Check sheet for the modelled part. Datum: model origin and axes. Units: mm. Round coordinates to 2 decimals unless told otherwise and drop trailing zeros. Write each loop counter-clockwise with the first axis right and the second up, starting at its lowest first coordinate (ties: lowest second). Pieces come first, ordered by that corner, then holes. Notation, with made-up numbers: M 0.5,23 L 12.5,23 A37 ccw 12.5,60 Z; hole C -36,12.25 d9. An arc over 180 degrees is marked long. One line per item, written item: value.
from build123d import *

# Parameters (mm, degrees)
SKETCH1_R           = 1.483161667
BOSS_EXTRUDE1_DEPTH = 88.9
FILLET1_R           = 2.54


with BuildPart() as part:
    # Sketch1 → Boss-Extrude1 (new body)
    with BuildSketch(Plane.XY):
        Polygon((6.273667096, -0.450919823), (2.607492887, 5.899080177), (-4.724855532, 5.899080177), (-8.391029741, -0.450919823), (-4.724855532, -6.800919823), (2.607492887, -6.800919823), align=None)
        with Locations((-1.058681322, -0.450919823)):
            Circle(SKETCH1_R, mode=Mode.SUBTRACT)
    extrude(amount=BOSS_EXTRUDE1_DEPTH)

    # Fillet1
    fillet1_edges = [part.edges().sort_by_distance(p)[0] for p in [
        (2.607492887, -6.800919823, 44.45),
        (-4.724855532, -6.800919823, 44.45),
        (-8.391029741, -0.450919823, 44.45),
        (-4.724855532, 5.899080177, 44.45),
        (2.607492887, 5.899080177, 44.45),
        (6.273667096, -0.450919823, 44.45),
    ]]
    fillet(fillet1_edges, radius=FILLET1_R)


solid = part.part
Q1. Sectioned sample at B-B on z = 43. Enter the section's corners in (x, y).
Completed:
outline: M -7.66,-1.72 L -5.46,-5.53 A2.54 ccw -3.26,-6.8 L 1.14,-6.8 A2.54 ccw 3.34,-5.53 L 5.54,-1.72 A2.54 ccw 5.54,0.82 L 3.34,4.63 A2.54 ccw 1.14,5.9 L -3.26,5.9 A2.54 ccw -5.46,4.63 L -7.66,0.82 A2.54 ccw Z; hole C -1.06,-0.45 d2.97
Q2. Sectioned sample at D-D on x = 2.5. Enter the section's corners in (y, z), and give its area (3 significant figures).
Completed:
outline: M -6.41,0 L 5.5,0 L 5.5,88.9 L -6.41,88.9 Z
area: 1,060 mm^2
Q3. Depth check by flat-ended pin: P1, Ø2.5, axis at x = -1.06, y = -0.45, coming from the -Z side; P2, Ø1, axis at y = 1, z = 73.5, coming from the -X side; P3, Ø1.5, axis at y = -3, z = 10, coming from the +X side; P4, Ø1.5, axis at x = -6, y = -1.5, coming from the -Z side. Enter the tip coordinate at first touch or a pass-through.
Completed:
P1: through
P2: x = -7.81
P3: x = 5.23
P4: z = 0
Q4. Sectioned sample at A-A on x = -1.75. Enter the section's corners in (y, z), and give its area (3 significant figures).
Completed:
outline: M -6.8,0 L -1.76,0 L -1.76,88.9 L -6.8,88.9 Z; M 0.86,0 L 5.9,0 L 5.9,88.9 L 0.86,88.9 Z
area: 896 mm^2
Q5. Draft check along Y on faces 1 (the cylindrical face through (-4.51, 5.57, 45.07)), 2 (the flat face through (-1, -6.801, 44)), 3 (the cylindrical face through (-8, -0.43, 45.07)), 4 (the cylindrical face through (0.356, -0.005, 43.828)). Enter one of: pulls with the +Y half, pulls with the -Y half, needs draft (parallel to the pull), parting line crosses it, or undercut.
Completed:
face 1: pulls with the +Y half
face 2: pulls with the -Y half
face 3: parting line crosses it
face 4: undercut
Q6. Sectioned sample at C-C on y = -3.25. Enter the section's corners in (x, z).
Completed:
outline: M -6.77,0 L 4.66,0 L 4.66,88.9 L -6.77,88.9 Z
Q7. Scan lines: line 1 (Y direction, x = -1, z = 68); line 2 (X direction, y = 0, z = 17.5); line 3 (Y direction, x = -3.5, z = 34). Record each from-to range of solid material in increasing order. Write a range as [from, to].
Completed:
line 1: [-6.8, -1.93], [1.03, 5.9]
line 2: [-7.96, -2.47], [0.35, 5.84]
line 3: [-6.79, 5.89]
